Check sheet for the drawn part. Datum: minimum x, y, z corner. Units: mm. Round coordinates to 2 decimals unless told otherwise and drop trailing zeros. Write each loop counter-clockwise with the first axis right and the second up, starting at its lowest first coordinate (ties: lowest second). Pieces come first, ordered by that corner, then holes. Notation, with made-up numbers: (16, -5) - (70, -5) arc R27 ccw to (70, 26) - close; hole circle Ø3 at (55, 26). An arc over 180 degrees is marked (long way). Write each question's results on one line, items separated by ' | '.
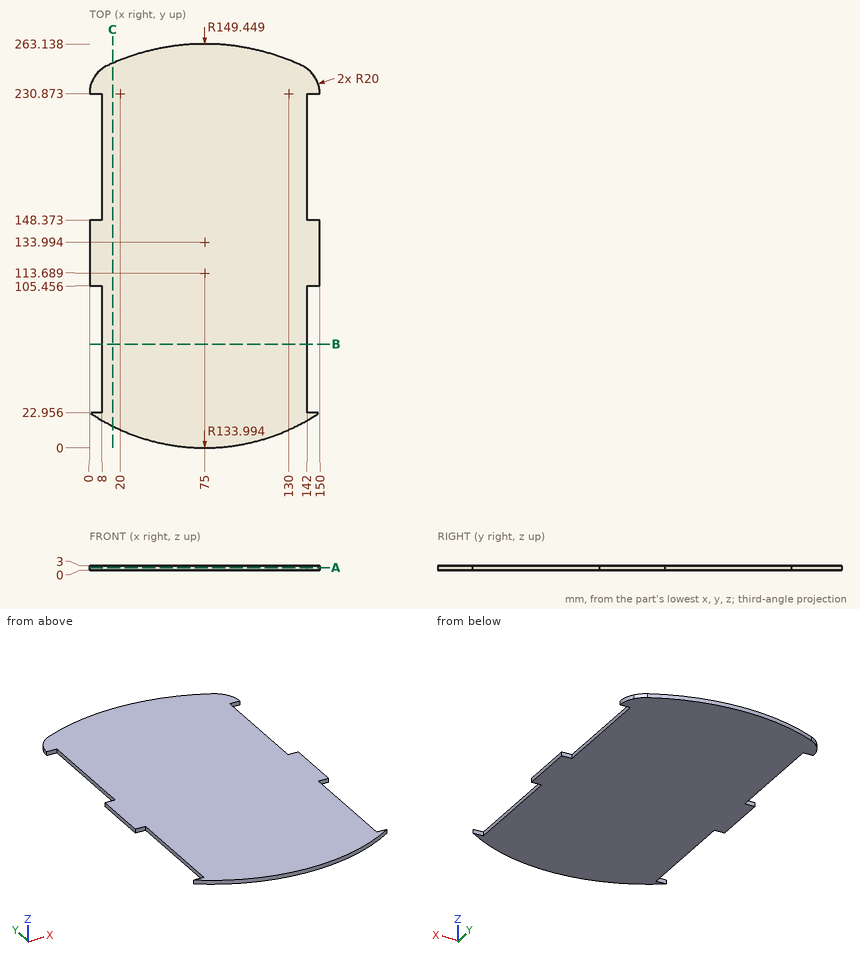
(1) Section check A-A (z = 1.8). Record the cut outline in (x, y), plus the area to 3 significant figures.
Answer:
outline: (0, 22.96) arc R133.99 ccw to (150, 22.96) - (142, 22.96) - (142, 105.46) - (150, 105.46) - (150, 148.37) - (142, 148.37) - (142, 230.87) - (150, 230.87) arc R20 ccw to (145.94, 242.96) arc R20 ccw to (138.5, 248.98) arc R149.45 ccw to (11.5, 248.98) arc R20 ccw to (4.06, 242.96) arc R20 ccw to (0, 230.87) - (8, 230.87) - (8, 148.37) - (0, 148.37) - (0, 105.46) - (8, 105.46) - (8, 22.96) - close | area: 34,700 mm2
(2) Section check C-C (x = 15). Record the cut outline in (y, z) (1 decimal).
Answer:
outline: (14.2, 0) - (250.6, 0) - (250.6, 3) - (14.2, 3) - close
(3) Thickness scan on L1, parallel to X at y = 64.5, z = 0.25; L2, parallel to Y at x = 143.5, z = 0.2 (1 decimal); L3, parallel to Y at x = 38.5, z = 1.3. Record the ranges inside material, lowest first.
Answer:
L1: 8 to 142 | L2: 18.8 to 23, 105.5 to 148.4, 230.9 to 245.6 | L3: 5.07 to 258.61
(4) Go/stop test with flat-tipped pins: pin 1 Ø0.9 at (x, z) = (144.5, 1) entering from +Y; pin 2 Ø0.9 at (x, z) = (147.5, 1) entering from +Y; pin 3 Ø0.9 at (x, z) = (147.5, 2) entering from -Y. Record where each tip stops, or that it passes through.
Answer:
pin 1: y = 245.11 | pin 2: y = 241.33 | pin 3: y = 21.02
(5) Section check B-B (y = 67.5). Record the cut outline in (x, z).
Answer:
outline: (8, 0) - (142, 0) - (142, 3) - (8, 3) - close
